from build123d import *

# Parameters (mm, degrees)
F0_R     = 2.95
F0_R_2   = 2.2
F0_R_3   = 1.425
F1_DEPTH = 3
F2_DEPTH = 1
F3_R     = 1.425
F4_DEPTH = 2


with BuildPart() as f1:
    # F0 (on Top) → F1 (new body)
    with BuildSketch(Plane.XY):
        with BuildLine():
            Line((3.95, -19.301667), (3.95, 0))
            Line((3.95, 0), (3.95, 19.301667))
            ThreePointArc((3.95, 19.301667), (3.106386, 21.387332), (1.05, 22.3))
            Line((1.05, 22.3), (-6.85, 22.3))
            ThreePointArc((-6.85, 22.3), (-8.97132, 21.42132), (-9.85, 19.3))
            Line((-9.85, 19.3), (-9.85, 0))
            Line((-9.85, 0), (-9.85, -19.3))
            ThreePointArc((-9.85, -19.3), (-8.97132, -21.42132), (-6.85, -22.3))
            Line((-6.85, -22.3), (1.05, -22.3))
            ThreePointArc((1.05, -22.3), (3.106386, -21.387332), (3.95, -19.301667))
        make_face()
        with Locations((-5.9, -18.35)):
            Circle(F0_R, mode=Mode.SUBTRACT)
        with Locations((-5.9, -12.35)):
            Circle(F0_R, mode=Mode.SUBTRACT)
        with Locations((-5.9, -6.35)):
            Circle(F0_R, mode=Mode.SUBTRACT)
        Polygon((0.082537, 1.761952), (0.117164, -1.701977), (-2.865373, -3.463929), (-5.882537, -1.761952), (-5.917164, 1.701977), (-2.934627, 3.463929), align=None, mode=Mode.SUBTRACT)
        with Locations((0, 6.35)):
            Circle(F0_R, mode=Mode.SUBTRACT)
        with Locations((0, 12.35)):
            Circle(F0_R, mode=Mode.SUBTRACT)
        with Locations((0, 18.35)):
            Circle(F0_R, mode=Mode.SUBTRACT)
        with Locations((0, 18.35)):
            Circle(F0_R)
        with Locations((0, 18.35)):
            Circle(F0_R_2, mode=Mode.SUBTRACT)
        with Locations((0, 12.35)):
            Circle(F0_R)
        with Locations((0, 12.35)):
            Circle(F0_R_2, mode=Mode.SUBTRACT)
        Polygon((-2.865373, -3.463929), (0.117164, -1.701977), (0.082537, 1.761952), (-2.934627, 3.463929), (-5.917164, 1.701977), (-5.882537, -1.761952), align=None)
        with Locations((-2.9, 0)):
            Circle(F0_R_3, mode=Mode.SUBTRACT)
        with Locations((-5.9, -6.35)):
            Circle(F0_R)
        with Locations((-5.9, -6.35)):
            Circle(F0_R_2, mode=Mode.SUBTRACT)
        with Locations((-5.9, -12.35)):
            Circle(F0_R)
        with Locations((-5.9, -12.35)):
            Circle(F0_R_2, mode=Mode.SUBTRACT)
        with Locations((-5.9, -18.35)):
            Circle(F0_R)
        with Locations((-5.9, -18.35)):
            Circle(F0_R_2, mode=Mode.SUBTRACT)
        with Locations((0, 6.35)):
            Circle(F0_R)
        with Locations((0, 6.35)):
            Circle(F0_R_2, mode=Mode.SUBTRACT)
    extrude(amount=-F1_DEPTH)

    # F0 (on Top) → F2 (cut)
    with BuildSketch(Plane.XY):
        with Locations((-5.9, -6.35)):
            Circle(F0_R)
        with Locations((-5.9, -6.35)):
            Circle(F0_R_2, mode=Mode.SUBTRACT)
        with Locations((-5.9, -12.35)):
            Circle(F0_R)
        with Locations((-5.9, -12.35)):
            Circle(F0_R_2, mode=Mode.SUBTRACT)
        with Locations((-5.9, -18.35)):
            Circle(F0_R)
        with Locations((-5.9, -18.35)):
            Circle(F0_R_2, mode=Mode.SUBTRACT)
        with Locations((0, 18.35)):
            Circle(F0_R)
        with Locations((0, 18.35)):
            Circle(F0_R_2, mode=Mode.SUBTRACT)
        with Locations((0, 12.35)):
            Circle(F0_R)
        with Locations((0, 12.35)):
            Circle(F0_R_2, mode=Mode.SUBTRACT)
        with Locations((0, 6.35)):
            Circle(F0_R)
        with Locations((0, 6.35)):
            Circle(F0_R_2, mode=Mode.SUBTRACT)
    extrude(amount=-F2_DEPTH, mode=Mode.SUBTRACT)

    # F3 (on face) → F4 (cut)
    with BuildSketch(Plane(origin=(0, 0, -3), x_dir=(1, 0, 0), z_dir=(0, 0, -1))):
        Polygon((-2.890558, -3.464089), (0.10471, -1.723868), (0.095268, 1.740221), (-2.909442, 3.464089), (-5.90471, 1.723868), (-5.895268, -1.740221), align=None)
        with Locations((-2.9, 0)):
            Circle(F3_R, mode=Mode.SUBTRACT)
    extrude(amount=-F4_DEPTH, mode=Mode.SUBTRACT)


solid = f1.part
Geometry check sheet. Reference: the model listing, model coordinates, mm. A direction names the side the tool comes from. Coordinates: 2 decimals unless noted, no trailing zeros. Write each loop counter-clockwise with the first axis right and the second up, starting at its lowest first coordinate (ties: lowest second). Pieces come first, ordered by that corner, then holes. Notation, with made-up numbers: (35, 54) -> (40, 54) arc R19 cw to (40, 66) -> close; hole circle Ø11 at (10.25, 4.25). An arc over 180 degrees is marked (long way). One line per question, with ' | ' between items.
1. Draft check along X on faces 1 (the flat face through (-1.4, -2.6, -2)), 2 (the flat face through (-9.85, 0, -1)), 3 (the flat face through (3.95, 0, -1)). Enter one of: +X half, -X half, draft (parallel to the pull), parting line (faces both ways), or undercut.
Answers:
face 1: undercut | face 2: -X half | face 3: +X half
2. Cross-section at C-C on y = -8. Record the cut outline in (x, z), and give its area (3 significant figures).
Answers:
outline: (-9.85, -3) -> (-7.36, -3) -> (-7.36, -1) -> (-8.35, -1) -> (-8.35, 0) -> (-9.85, 0) -> close; (-4.44, -3) -> (3.95, -3) -> (3.95, 0) -> (-3.45, 0) -> (-3.45, -1) -> (-4.44, -1) -> close | area: 30.7 mm²
3. Cross-section at A-A on y = 18.35. Record the cut outline in (x, z).
Answers:
outline: (-9.85, -3) -> (-2.2, -3) -> (-2.2, -1) -> (-2.95, -1) -> (-2.95, 0) -> (-9.85, 0) -> close; (2.2, -3) -> (3.95, -3) -> (3.95, 0) -> (2.95, 0) -> (2.95, -1) -> (2.2, -1) -> close
4. Cross-section at B-B on z = -2.45. Record the cut outline in (x, y), and give its area (3 significant figures).
Answers:
outline: (-9.85, -19.3) arc R3 ccw to (-6.85, -22.3) -> (1.05, -22.3) arc R3 ccw to (3.95, -19.3) -> (3.95, 19.3) arc R3 ccw to (1.05, 22.3) -> (-6.85, 22.3) arc R3 ccw to (-9.85, 19.3) -> close; hole circle Ø4.4 at (-5.9, -18.35); hole circle Ø4.4 at (-5.9, -12.35); hole circle Ø4.4 at (-5.9, -6.35); hole (-5.9, -1.72) -> (-2.91, -3.46) -> (0.1, -1.74) -> (0.1, 1.72) -> (-2.89, 3.46) -> (-5.9, 1.74) -> close; hole circle Ø4.4 at (0, 6.35); hole circle Ø4.4 at (0, 12.35); hole circle Ø4.4 at (0, 18.35) | area: 485 mm²
5. Thickness scan on probe 1 along Y at (x, z) = (-1, -2.7); probe 2 along Y at (x, z) = (-6.75, -0.2); probe 3 along Y at (x, z) = (1.75, -0.7). Record the ranges inside material, lowest first. Write a range as from..to.
Answers:
probe 1: y = -22.3..-2.37, 2.37..4.39, 8.31..10.39, 14.31..16.39, 20.31..22.3 | probe 2: y = -22.3..-21.17, -15.53..-15.17, -9.53..-9.17, -3.53..22.3 | probe 3: y = -22.19..3.98, 8.72..9.98, 14.72..15.98, 20.72..22.19
6. Depth check by flat-ended pin: pin 1 Ø7 at (x, y) = (0, 12.35) entering from +Z; pin 2 Ø2.5 at (x, y) = (0, 6.35) entering from -Z; pin 3 Ø4.5 at (x, y) = (0, 6.35) entering from +Z; pin 4 Ø1.8 at (x, y) = (-3.5, -1.5) entering from -Z. Enter the tip coordinate at first touch or a pass-through.
Answers:
pin 1: stops at z = 0 | pin 2: passes through | pin 3: stops at z = -1 | pin 4: stops at z = -1
7. Cross-section at D-D on y = -2.5. Record the cut outline in (x, z), and give its area (3 significant figures).
Answers:
outline: (-9.85, -3) -> (-4.57, -3) -> (-4.57, -1) -> (-1.23, -1) -> (-1.23, -3) -> (3.95, -3) -> (3.95, 0) -> (-9.85, 0) -> close | area: 34.7 mm²
8. Set-up check for faces 4 (the flat face through (-4.4, -2.6, -2)), 5 (the flat face through (-1, 4, -1)), 6 (the cylindrical face through (-0.477, 4.202, -1.986)): record each of +Z, -Z, +X, -X, +Y, -Y from which the full face is reachable in a straight line by a thin tool's end or side.
Answers:
face 4: -Z | face 5: +Z | face 6: +Z, -Z
